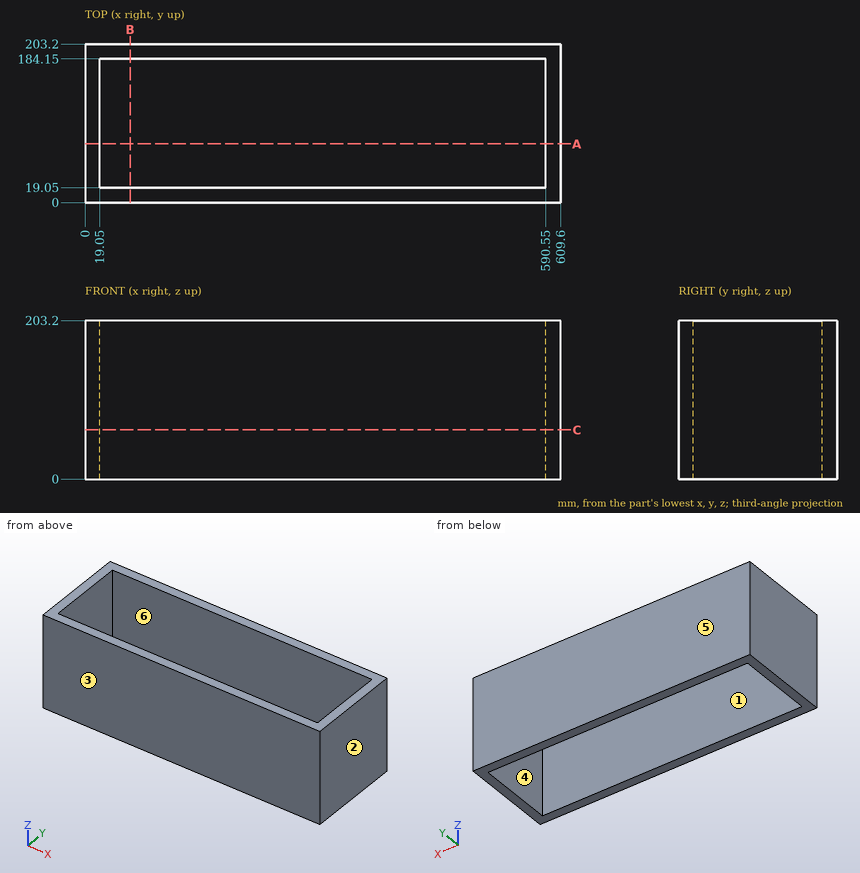
Answer from the drawing. Dimensions are ordinates in mm from the lowest x, y and z of the part. A direction names the side the tool comes from. Round coordinates to 2 decimals unless told otherwise and drop trailing zeros. Order: outer loops, then holes, each group sorted by start corner. A loop starts at its lowest first (then second) coordinate and runs counter-clockwise, first axis right, second up. Notation, with made-up numbers: (60, -16.5) - (86, -16.5) arc R25 cw to (86, -0.5) - close; hole circle Ø3 at (67, 50). An arc over 180 degrees is marked (long way). Put each result on its own line as item: value. Start each with the question number.
(1) For the marked faces 5 and 6, determine the directions among +Z, -Z, +X, -X, +Y, -Y from which every point of the face is accessible in a straight line to the end or side of a thin tool.
(2) Find section C-C (z = 63). Give the vertices of the cut face in (x, y).
(3) Determine the mould class of the marked faces 1, 2, 3 and 4 for opening direction X: released by +X, released by -X, zero draft, split by the parting line, or undercut.
(4) Straight lines are drawn through the part: probe 1 along X at (y, z) = (154.5, 145.5); probe 2 along Y at (x, z) = (514, 113.5). For each, find the intervals that lie inside material, in ascending order. Write a range as from..to.
(5) Find section A-A (y = 75). Give the vertices of the cut face in (x, z), plus the area to 3 significant figures.
(6) Find section B-B (x = 58). Give the vertices of the cut face in (y, z).
Reply:
1. face 5: +Z, -Z, +X, -X, +Y
1. face 6: +Z, -Z
2. outline: (0, 0) - (609.6, 0) - (609.6, 203.2) - (0, 203.2) - close; hole (19.05, 19.05) - (590.55, 19.05) - (590.55, 184.15) - (19.05, 184.15) - close
3. face 1: undercut
3. face 2: released by +X
3. face 3: zero draft
3. face 4: undercut
4. probe 1: 0..19.05, 590.55..609.6
4. probe 2: 0..19.05, 184.15..203.2
5. outline: (0, 0) - (19.05, 0) - (19.05, 203.2) - (0, 203.2) - close; (590.55, 0) - (609.6, 0) - (609.6, 203.2) - (590.55, 203.2) - close
5. area: 7,740 mm^2
6. outline: (0, 0) - (19.05, 0) - (19.05, 203.2) - (0, 203.2) - close; (184.15, 0) - (203.2, 0) - (203.2, 203.2) - (184.15, 203.2) - close
